```python
from build123d import *

# Parameters (mm, degrees)
SKETCH_W        = 101.75
SKETCH_H        = 25.4
PAD_DEPTH       = 4
FILLET_R        = 1
FILLET001_R     = 1
FILLET002_R     = 1
FILLET003_R     = 1
SKETCH001_W     = 90.9
SKETCH001_H     = 4.6
POCKET_DEPTH    = 5
CHAMFER_SIZE    = 1
CHAMFER001_SIZE = 1
CHAMFER002_SIZE = 1
CHAMFER003_SIZE = 1
SKETCH002_W     = 5.2
SKETCH002_H     = 2
POCKET001_DEPTH = 5
SKETCH003_W     = 50
SKETCH003_H     = 6
POCKET002_DEPTH = 5
SKETCH004_W     = 10.6
SKETCH004_H     = 4.6
POCKET003_DEPTH = 5
SKETCH005_W     = 35
SKETCH005_H     = 12.5
POCKET004_DEPTH = 2.5
CHAMFER004_SIZE = 2.49
CHAMFER005_SIZE = 0.74
CHAMFER006_SIZE = 0.63
CHAMFER007_SIZE = 0.63
CHAMFER008_SIZE = 0.74
CHAMFER009_SIZE = 2.49
SKETCH006_W     = 1
SKETCH006_H     = 5.6
PAD001_DEPTH    = 10
SKETCH007_W     = 3
SKETCH007_H     = 3
PAD002_DEPTH    = 0.75
CHAMFER010_SIZE = 1
SKETCH008_W     = 1
SKETCH008_H     = 5.6
PAD003_DEPTH    = 10
SKETCH009_W     = 3
SKETCH009_H     = 3
PAD004_DEPTH    = 0.75
CHAMFER011_SIZE = 3
CHAMFER012_SIZE = 1
SKETCH010_W     = 1
SKETCH010_H     = 5.6
PAD005_DEPTH    = 10
SKETCH011_W     = 3
SKETCH011_H     = 3
PAD006_DEPTH    = 0.75
CHAMFER013_SIZE = 1
SKETCH012_W     = 1
SKETCH012_H     = 5.6
PAD007_DEPTH    = 10
SKETCH013_W     = 3
SKETCH013_H     = 3
PAD008_DEPTH    = 0.75
CHAMFER014_SIZE = 2
CHAMFER015_SIZE = 1
SKETCH014_W     = 95.5
SKETCH014_H     = 9.5
POCKET005_DEPTH = 1
SKETCH015_R     = 2
PAD009_DEPTH    = 2
SKETCH016_R     = 1.05
POCKET006_DEPTH = 5
SKETCH017_R     = 2
PAD010_DEPTH    = 2
SKETCH018_R     = 1.05
POCKET007_DEPTH = 5
SKETCH019_R     = 2
POCKET008_DEPTH = 2
SKETCH020_R     = 2
POCKET009_DEPTH = 2
SKETCH022_W     = 8.5
SKETCH022_H     = 0.85
POCKET011_DEPTH = 2.5
SKETCH023_W     = 16
SKETCH023_H     = 6
POCKET012_DEPTH = 2.5
SKETCH024_W     = 12.75
SKETCH024_H     = 6.5
POCKET013_DEPTH = 2.5


with BuildPart() as part:
    # Sketch → Pad (new body)
    with BuildSketch(Plane.XZ):
        with Locations((50.875, 12.7)):
            Rectangle(SKETCH_W, SKETCH_H)
    extrude(amount=PAD_DEPTH)

    # Fillet
    fillet_edges = [part.edges().sort_by_distance(p)[0] for p in [
        (101.75, -2, 0),
    ]]
    fillet(fillet_edges, radius=FILLET_R)

    # Fillet001
    fillet001_edges = [part.edges().sort_by_distance(p)[0] for p in [
        (101.75, -2, 25.4),
    ]]
    fillet(fillet001_edges, radius=FILLET001_R)

    # Fillet002
    fillet002_edges = [part.edges().sort_by_distance(p)[0] for p in [
        (0, -2, 25.4),
    ]]
    fillet(fillet002_edges, radius=FILLET002_R)

    # Fillet003
    fillet003_edges = [part.edges().sort_by_distance(p)[0] for p in [
        (0, -2, 0),
    ]]
    fillet(fillet003_edges, radius=FILLET003_R)

    # Sketch001 (on Face10 of Fillet003) → Pocket (cut)
    with BuildSketch(Plane.XZ.offset(4)):
        with Locations((50.95, 11.95)):
            Rectangle(SKETCH001_W, SKETCH001_H)
    extrude(amount=-POCKET_DEPTH, mode=Mode.SUBTRACT)

    # Chamfer
    chamfer_edges = [part.edges().sort_by_distance(p)[0] for p in [
        (50.95, -4, 14.25),
    ]]
    chamfer(chamfer_edges, length=CHAMFER_SIZE)

    # Chamfer001
    chamfer001_edges = [part.edges().sort_by_distance(p)[0] for p in [
        (5.5, -4, 11.95),
    ]]
    chamfer(chamfer001_edges, length=CHAMFER001_SIZE)

    # Chamfer002
    chamfer002_edges = [part.edges().sort_by_distance(p)[0] for p in [
        (50.45, -4, 9.65),
    ]]
    chamfer(chamfer002_edges, length=CHAMFER002_SIZE)

    # Chamfer003
    chamfer003_edges = [part.edges().sort_by_distance(p)[0] for p in [
        (96.4, -4, 12.45),
    ]]
    chamfer(chamfer003_edges, length=CHAMFER003_SIZE)

    # Sketch002 (on Face6 of Chamfer003) → Pocket001 (cut)
    with BuildSketch(Plane.XZ.offset(4)):
        with Locations((20.3, 3)):
            Rectangle(SKETCH002_W, SKETCH002_H)
    extrude(amount=-POCKET001_DEPTH, mode=Mode.SUBTRACT)

    # Sketch003 (on Face7 of Pocket001) → Pocket002 (cut)
    with BuildSketch(Plane.XZ.offset(4)):
        with Locations((50.7, 12)):
            Rectangle(SKETCH003_W, SKETCH003_H)
    extrude(amount=-POCKET002_DEPTH, mode=Mode.SUBTRACT)

    # Sketch004 (on Face7 of Pocket002) → Pocket003 (cut)
    with BuildSketch(Plane.XZ.offset(4)):
        with Locations((80.9, 4)):
            Rectangle(SKETCH004_W, SKETCH004_H)
    extrude(amount=-POCKET003_DEPTH, mode=Mode.SUBTRACT)

    # Sketch005 (on Face7 of Pocket003) → Pocket004 (cut)
    with BuildSketch(Plane.XZ.offset(4)):
        with Locations((51, 10.95)):
            Rectangle(SKETCH005_W, SKETCH005_H)
    extrude(amount=-POCKET004_DEPTH, mode=Mode.SUBTRACT)

    # Chamfer004
    chamfer004_edges = [part.edges().sort_by_distance(p)[0] for p in [
        (51, -4, 4.7),
    ]]
    chamfer(chamfer004_edges, length=CHAMFER004_SIZE)

    # Chamfer005
    chamfer005_edges = [part.edges().sort_by_distance(p)[0] for p in [
        (25.7, -1.5, 14.25),
    ]]
    chamfer(chamfer005_edges, length=CHAMFER005_SIZE)

    # Chamfer006
    chamfer006_edges = [part.edges().sort_by_distance(p)[0] for p in [
        (25.7, -1.5, 9.65),
    ]]
    chamfer(chamfer006_edges, length=CHAMFER006_SIZE)

    # Chamfer007
    chamfer007_edges = [part.edges().sort_by_distance(p)[0] for p in [
        (75.7, -1.5, 9.65),
    ]]
    chamfer(chamfer007_edges, length=CHAMFER007_SIZE)

    # Chamfer008
    chamfer008_edges = [part.edges().sort_by_distance(p)[0] for p in [
        (75.7, -1.5, 14.25),
    ]]
    chamfer(chamfer008_edges, length=CHAMFER008_SIZE)

    # Chamfer009
    chamfer009_edges = [part.edges().sort_by_distance(p)[0] for p in [
        (51, -4, 17.2),
    ]]
    chamfer(chamfer009_edges, length=CHAMFER009_SIZE)

    # Sketch006 (on Face34 of Chamfer009) → Pad001 (join)
    with BuildSketch(Plane(origin=(0, 0, 0), x_dir=(1, 0, 0), z_dir=(0, 1, 0))):
        with Locations((2.5, -4.3)):
            Rectangle(SKETCH006_W, SKETCH006_H)
    extrude(amount=PAD001_DEPTH)

    # Sketch007 (on Face51 of Pad001) → Pad002 (join)
    with BuildSketch(Plane(origin=(2, 0, 0), x_dir=(0, 0, -1), z_dir=(-1, 0, 0))):
        with Locations((-5, -8.5)):
            Rectangle(SKETCH007_W, SKETCH007_H)
    extrude(amount=PAD002_DEPTH)

    # Chamfer010
    chamfer010_edges = [part.edges().sort_by_distance(p)[0] for p in [
        (1.25, 10, 5),
    ]]
    chamfer(chamfer010_edges, length=CHAMFER010_SIZE)

    # Sketch008 (on Face4 of Chamfer010) → Pad003 (join)
    with BuildSketch(Plane(origin=(0, 0, 0), x_dir=(1, 0, 0), z_dir=(0, 1, 0))):
        with Locations((2.5, -14.8)):
            Rectangle(SKETCH008_W, SKETCH008_H)
    extrude(amount=PAD003_DEPTH)

    # Sketch009 (on Face24 of Pad003) → Pad004 (join)
    with BuildSketch(Plane(origin=(2, 0, 0), x_dir=(0, 0, -1), z_dir=(-1, 0, 0))):
        with Locations((-15, -8.5)):
            Rectangle(SKETCH009_W, SKETCH009_H)
    extrude(amount=PAD004_DEPTH)

    # Chamfer011
    chamfer011_edges = [part.edges().sort_by_distance(p)[0] for p in [
        (2.5, 10, 12),
    ]]
    chamfer(chamfer011_edges, length=CHAMFER011_SIZE)

    # Chamfer012
    chamfer012_edges = [part.edges().sort_by_distance(p)[0] for p in [
        (1.25, 10, 15.75),
    ]]
    chamfer(chamfer012_edges, length=CHAMFER012_SIZE)

    # Sketch010 (on Face7 of Chamfer012) → Pad005 (join)
    with BuildSketch(Plane(origin=(0, 0, 0), x_dir=(1, 0, 0), z_dir=(0, 1, 0))):
        with Locations((99.3, -4.8)):
            Rectangle(SKETCH010_W, SKETCH010_H)
    extrude(amount=PAD005_DEPTH)

    # Sketch011 (on Face35 of Pad005) → Pad006 (join)
    with BuildSketch(Plane(origin=(99.8, 0, 0), x_dir=(0, 0, 1), z_dir=(1, 0, 0))):
        with Locations((4.5, -8.5)):
            Rectangle(SKETCH011_W, SKETCH011_H)
    extrude(amount=PAD006_DEPTH)

    # Chamfer013
    chamfer013_edges = [part.edges().sort_by_distance(p)[0] for p in [
        (100.55, 10, 4.5),
    ]]
    chamfer(chamfer013_edges, length=CHAMFER013_SIZE)

    # Sketch012 (on Face4 of Chamfer013) → Pad007 (join)
    with BuildSketch(Plane(origin=(0, 0, 0), x_dir=(1, 0, 0), z_dir=(0, 1, 0))):
        with Locations((99.3, -14.8)):
            Rectangle(SKETCH012_W, SKETCH012_H)
    extrude(amount=PAD007_DEPTH)

    # Sketch013 (on Face54 of Pad007) → Pad008 (join)
    with BuildSketch(Plane(origin=(99.8, 0, 0), x_dir=(0, 0, 1), z_dir=(1, 0, 0))):
        with Locations((14.5, -8.5)):
            Rectangle(SKETCH013_W, SKETCH013_H)
    extrude(amount=PAD008_DEPTH)

    # Chamfer014
    chamfer014_edges = [part.edges().sort_by_distance(p)[0] for p in [
        (99.3, 10, 12),
    ]]
    chamfer(chamfer014_edges, length=CHAMFER014_SIZE)

    # Chamfer015
    chamfer015_edges = [part.edges().sort_by_distance(p)[0] for p in [
        (100.55, 10, 15),
    ]]
    chamfer(chamfer015_edges, length=CHAMFER015_SIZE)

    # Sketch014 (on Face11 of Chamfer015) → Pocket005 (cut)
    with BuildSketch(Plane(origin=(0, 0, 0), x_dir=(1, 0, 0), z_dir=(0, 1, 0))):
        with Locations((50.75, -13.25)):
            Rectangle(SKETCH014_W, SKETCH014_H)
    extrude(amount=-POCKET005_DEPTH, mode=Mode.SUBTRACT)

    # Sketch015 (on Face7 of Pocket005) → Pad009 (join)
    with BuildSketch(Plane(origin=(99.8, 0, 0), x_dir=(0, 0, 1), z_dir=(1, 0, 0))):
        with Locations((16.5, -1)):
            Circle(SKETCH015_R)
    extrude(amount=-PAD009_DEPTH)

    # Sketch016 (on Face98 of Pad009) → Pocket006 (cut)
    with BuildSketch(Plane(origin=(99.8, 0, 0), x_dir=(0, 0, 1), z_dir=(1, 0, 0))):
        with Locations((16.5, -1)):
            Circle(SKETCH016_R)
    extrude(amount=-POCKET006_DEPTH, mode=Mode.SUBTRACT)

    # Sketch017 (on Face39 of Pocket006) → Pad010 (join)
    with BuildSketch(Plane(origin=(2, 0, 0), x_dir=(0, 0, -1), z_dir=(-1, 0, 0))):
        with Locations((-16.5, -1)):
            Circle(SKETCH017_R)
    extrude(amount=-PAD010_DEPTH)

    # Sketch018 (on Face103 of Pad010) → Pocket007 (cut)
    with BuildSketch(Plane(origin=(2, 0, 0), x_dir=(0, 0, -1), z_dir=(-1, 0, 0))):
        with Locations((-16.5, -1)):
            Circle(SKETCH018_R)
    extrude(amount=-POCKET007_DEPTH, mode=Mode.SUBTRACT)

    # Sketch019 (on Face18 of Pocket007) → Pocket008 (cut)
    with BuildSketch(Plane(origin=(0, 0, 0), x_dir=(0, 0, -1), z_dir=(-1, 0, 0))):
        with Locations((-16.5, -1)):
            Circle(SKETCH019_R)
    extrude(amount=-POCKET008_DEPTH, mode=Mode.SUBTRACT)

    # Sketch020 (on Face29 of Pocket008) → Pocket009 (cut)
    with BuildSketch(Plane(origin=(101.75, 0, 0), x_dir=(0, 0, 1), z_dir=(1, 0, 0))):
        with Locations((16.5, -1)):
            Circle(SKETCH020_R)
    extrude(amount=-POCKET009_DEPTH, mode=Mode.SUBTRACT)

    # Sketch022 → Pocket011 (cut)
    with BuildSketch(Plane(origin=(0, 0, 0), x_dir=(1, 0, 0), z_dir=(0, 1, 0))):
        with Locations((20.25, -1.075)):
            Rectangle(SKETCH022_W, SKETCH022_H)
    extrude(amount=-POCKET011_DEPTH, mode=Mode.SUBTRACT)

    # Sketch023 (on Face10 of Pocket011) → Pocket012 (cut)
    with BuildSketch(Plane(origin=(0, 0, 0), x_dir=(1, 0, 0), z_dir=(0, 1, 0))):
        with Locations((20, -4.5)):
            Rectangle(SKETCH023_W, SKETCH023_H)
    extrude(amount=-POCKET012_DEPTH, mode=Mode.SUBTRACT)

    # Sketch024 (on Face10 of Pocket012) → Pocket013 (cut)
    with BuildSketch(Plane(origin=(0, 0, 0), x_dir=(1, 0, 0), z_dir=(0, 1, 0))):
        with Locations((80.875, -4.05)):
            Rectangle(SKETCH024_W, SKETCH024_H)
    extrude(amount=-POCKET013_DEPTH, mode=Mode.SUBTRACT)


solid = part.part
```
Design review of the part built by this model. Coordinates are the model's own, in mm. A direction names the side the tool comes from. Round coordinates to 2 decimals unless told otherwise and drop trailing zeros. Order: outer loops, then holes, each group sorted by start corner. A loop starts at its lowest first (then second) coordinate and runs counter-clockwise, first axis right, second up. Notation, with made-up numbers: (39, 55) - (89, 55) arc R14 ccw to (89, 74) - close; hole circle Ø3 at (51.5, 30.25). An arc over 180 degrees is marked (long way). Return JSON: item names as keys, results as strings.
Q1. For pin 1 Ø1.7 at (y, z) = (3.5, 4.5) entering from +X; pin 2 Ø3 at (y, z) = (6.5, 8) entering from -X; pin 3 Ø10 at (x, z) = (88, 14) entering from +Y; pin 4 Ø4.5 at (y, z) = (1, 15.5) entering from -X, all flat-tipped, find the tip position at first contact; note any pin that passes through.
Computed values:
{"pin 1": "stops at x = 99.8", "pin 2": "stops at x = 2", "pin 3": "stops at y = 0", "pin 4": "stops at x = 0"}
Q2. Consider section A-A on y = 1. Give the number of separate pieces and of enclosed holes in the cut face, plus the area to 3 significant figures.
Computed values:
{"separate pieces": "6", "enclosed holes": "0", "area": "23.7 mm2"}
Q3. Machinability: for faces 1 (the flat face through (26, -1, 1.5)), 2 (the flat face through (2, 9, 14)), 3 (the flat face through (50.76, -2.74, 3.47)), 4 (the cylindrical face through (3.21, 2.56, 17.75)), which of the approach directions +Z, -Z, +X, -X, +Y, -Y give a long, thin tool a straight path to every point of the face, cutting with its end or side? Answer none if there is none.
Computed values:
{"face 1": "+Y", "face 2": "-X, +Y", "face 3": "-Y", "face 4": "none"}
Q4. Wall thickness on L1, parallel to Z at x = 3.4, y = 1; L2, parallel to Z at x = 99.4, y = 1; L3, parallel to X at y = 6.75, z = 6: over which ranges is each line inside the solid? List them lowest first. Write a range as [from, to].
Computed values:
{"L1": "z = [14.5, 15.45], [17.55, 18.5]", "L2": "z = [2, 7.6], [12, 15.45], [17.55, 18.5]", "L3": "x = [2, 3], [98.8, 99.8]"}
Q5. Consider section C-C on x = 31.5. Write out the cut boundary in (y, z).
Computed values:
{"outline": "(-4, 0) - (0, 0) - (0, 8.5) - (-1, 8.5) - (-1, 9) - (-3.65, 9) - (-4, 8.65) - close; (-4, 15.25) - (-3.75, 15) - (-1, 15) - (-1, 18) - (0, 18) - (0, 25.4) - (-4, 25.4) - close"}
Q6. The part is to be moulded in two halves that separate along X. For faces 5 (the flat face through (51, -1.5, 16)), 6 (the flat face through (50, -2, 25.4)), 7 (the flat face through (50.4, -1.2, 9)), say which applies: pulls with the +X half, pulls with the -X half, needs draft (parallel to the pull), parting line crosses it, or undercut.
Computed values:
{"face 5": "undercut", "face 6": "needs draft", "face 7": "undercut"}
